from build123d import *

# Parameters (mm, degrees)
SALIENTE_EXTRUIR1_DEPTH  = 12
CROQUIS2_W               = 12.5
CROQUIS2_H               = 16.5
CROQUIS2_W_2             = 9.5
CROQUIS2_H_2             = 13.5
SALIENTE_EXTRUIR2_DEPTH  = 2
SALIENTE_EXTRUIR4_DEPTH  = 11
CROQUIS4_R               = 1.6
CORTAR_EXTRUIR1_DEPTH    = 2.5
CROQUIS5_W               = 17.29289048
CROQUIS5_H               = 2.276098228
CROQUIS5_W_2             = 23.449996424
CROQUIS5_H_2             = 5.821617307
CORTAR_EXTRUIR2_DEPTH    = 2
SALIENTE_EXTRUIR5_DEPTH  = 3
CROQUIS7_W               = 60
CROQUIS7_H               = 12
SALIENTE_EXTRUIR6_DEPTH  = 3
CORTAR_EXTRUIR3_DEPTH    = 42
VACIADO4_START           = -15.778481013
VACIADO4_DEPTH           = 39
VACIADO4_2_OUTLINE_W     = 28
VACIADO4_2_OUTLINE_H     = 9
VACIADO4_2_DEPTH         = 4
VACIADO4_START_2         = 19.221518987
VACIADO4_3_OUTLINE_W     = 28
VACIADO4_3_OUTLINE_H     = 9
VACIADO4_3_DEPTH         = 4
VACIADO4_START_3         = -3.938481013
VACIADO4_4_OUTLINE_W     = 9.5
VACIADO4_4_OUTLINE_H     = 1.5
VACIADO4_4_DEPTH         = 13.5
REDONDEO2_R              = 4
REDONDEO3_R              = 4
CROQUIS10_W              = 2.5
CROQUIS10_H              = 7
SALIENTE_EXTRUIR8_DEPTH  = 24
CROQUIS11_R              = 1.65
CORTAR_EXTRUIR4_DEPTH    = 2.5
CROQUIS14_R              = 1.6
SALIENTE_EXTRUIR10_DEPTH = 0.5
CROQUIS15_W              = 28.276285021
CROQUIS15_H              = 42
CORTAR_EXTRUIR5_DEPTH    = 12
CROQUIS16_W              = 42
CROQUIS16_H              = 12
SALIENTE_EXTRUIR11_DEPTH = 2
CORTAR_EXTRUIR6_DEPTH    = 2.5
CROQUIS19_W              = 18.223714979
CROQUIS19_H              = 1.5
SALIENTE_EXTRUIR16_DEPTH = 9
REDONDEO4_R              = 2
REDONDEO5_R              = 2
REDONDEO6_R              = 2


with BuildPart() as part:
    # Croquis1 → Saliente-Extruir1 (new body)
    with BuildSketch(Plane(origin=(0, 0, 0), x_dir=(1, 0, 0), z_dir=(0, 1, 0))):
        Polygon((30.683544304, -17.721518987), (30.683544304, -21.721518987), (-29.316455696, -21.721518987), (-29.316455696, 14.278481013), (30.683544304, 14.278481013), (30.683544304, 10.278481013), (2.683544304, 10.278481013), (2.683544304, -17.721518987), align=None)
    extrude(amount=SALIENTE_EXTRUIR1_DEPTH)

    # Croquis2 → Saliente-Extruir2 (add)
    with BuildSketch(Plane(origin=(0, 12, 0), x_dir=(1, 0, 0), z_dir=(0, 1, 0))):
        with Locations((-21.066455696, -2.811518987)):
            Rectangle(CROQUIS2_W, CROQUIS2_H)
        with Locations((-21.066455696, -2.811518987)):
            Rectangle(CROQUIS2_W_2, CROQUIS2_H_2, mode=Mode.SUBTRACT)
    extrude(amount=SALIENTE_EXTRUIR2_DEPTH)

    # Croquis3 → Saliente-Extruir4 (add)
    with BuildSketch(Plane(origin=(0, 12, 0), x_dir=(1, 0, 0), z_dir=(0, 1, 0))):
        Polygon((-7.816455696, -12.741518987), (-7.816455696, -41.560532566), (-7.816455696, -45.664219129), (-9.816455696, -45.664219129), (-9.816455696, -41.560532566), (-9.816455696, -12.741518987), align=None)
    extrude(amount=SALIENTE_EXTRUIR4_DEPTH)

    # Croquis4 → Cortar-Extruir1 (cut)
    with BuildSketch(Plane.ZY.offset(9.816455696)):
        with Locations((40.551518987, 19.507537468)):
            Circle(CROQUIS4_R)
    extrude(amount=-CORTAR_EXTRUIR1_DEPTH, mode=Mode.SUBTRACT)

    # Croquis5 → Cortar-Extruir2 (cut)
    with BuildSketch(Plane.ZY.offset(9.816455696)):
        with Locations((37.017773889, 13.138049114)):
            Rectangle(CROQUIS5_W, CROQUIS5_H)
        with Locations((24.466517199, 20.089191347)):
            Rectangle(CROQUIS5_W_2, CROQUIS5_H_2)
    extrude(amount=-CORTAR_EXTRUIR2_DEPTH, mode=Mode.SUBTRACT)

    # Croquis6 → Saliente-Extruir5 (add)
    with BuildSketch(Plane.XY.offset(21.721518987)):
        Polygon((-29.316455696, 0), (30.683544304, 0), (30.683544304, 12), (-7.816455696, 12), (-9.816455696, 12), (-29.316455696, 12), align=None)
    extrude(amount=SALIENTE_EXTRUIR5_DEPTH)

    # Croquis7 → Saliente-Extruir6 (add)
    with BuildSketch(Plane(origin=(0, 0, -14.278481013), x_dir=(-1, 0, 0), z_dir=(0, 0, -1))):
        with Locations((-0.683544304, 6)):
            Rectangle(CROQUIS7_W, CROQUIS7_H)
    extrude(amount=SALIENTE_EXTRUIR6_DEPTH)

    # Croquis8 → Cortar-Extruir3 (cut)
    with BuildSketch(Plane.XY.offset(24.721518987)):
        with BuildLine():
            Line((-29.316455696, 0), (-18.316455696, 0))
            ThreePointArc((-18.316455696, 0), (-26.094630289, 3.221825407), (-29.316455696, 11))
            Line((-29.316455696, 11), (-29.316455696, 0))
        make_face()
    extrude(amount=-CORTAR_EXTRUIR3_DEPTH, mode=Mode.SUBTRACT)

    # Vaciado4: read off the stored shape, not the designer's step
    # Vaciado4 outline → Vaciado4 (cut)
    with BuildSketch(Plane.XY.offset(VACIADO4_START)):
        with BuildLine():
            Line((1.183544304, 10.5), (-27.803288677, 10.5))
            ThreePointArc((-27.803288677, 10.5), (-24.854804112, 4.107975624), (-18.316455696, 1.5))
            Line((-18.316455696, 1.5), (1.183544304, 1.5))
            Line((1.183544304, 1.5), (1.183544304, 10.5))
        make_face()
    extrude(amount=VACIADO4_DEPTH, mode=Mode.SUBTRACT)

    # Vaciado4 2 outline → Vaciado4 2 (cut)
    with BuildSketch(Plane.XY.offset(VACIADO4_START)):
        with Locations((15.183544304, 6)):
            Rectangle(VACIADO4_2_OUTLINE_W, VACIADO4_2_OUTLINE_H)
    extrude(amount=VACIADO4_2_DEPTH, mode=Mode.SUBTRACT)

    # Vaciado4 3 outline → Vaciado4 3 (cut)
    with BuildSketch(Plane.XY.offset(VACIADO4_START_2)):
        with Locations((15.183544304, 6)):
            Rectangle(VACIADO4_3_OUTLINE_W, VACIADO4_3_OUTLINE_H)
    extrude(amount=VACIADO4_3_DEPTH, mode=Mode.SUBTRACT)

    # Vaciado4 4 outline → Vaciado4 4 (cut)
    with BuildSketch(Plane.XY.offset(VACIADO4_START_3)):
        with Locations((-21.066455696, 11.25)):
            Rectangle(VACIADO4_4_OUTLINE_W, VACIADO4_4_OUTLINE_H)
    extrude(amount=VACIADO4_4_DEPTH, mode=Mode.SUBTRACT)

    # Redondeo2
    # the kernel refuses this fillet: 4 mm, written as the material it adds along each edge
    with BuildSketch(Plane(origin=(-9.816455696, 12, 24.721518987), x_dir=(0, -1, 0), z_dir=(1, 0, 0))) as redondeo2_piece_1:
        with BuildLine():
            CenterArc((3.984641355, -4), REDONDEO2_R, 90, 84.977462971)
            Line((0, -3.649809662), (0, 0))
            Line((0, 0), (3.984641355, 0))
        make_face()
    extrude(amount=2)
    with BuildSketch(Plane(origin=(-9.816455696, 14.276098228, 28.371328649), x_dir=(0, 0, 1), z_dir=(1, 0, 0))) as redondeo2_piece_2:
        with BuildLine():
            CenterArc((3.609454623, 4), REDONDEO2_R, 205.52948015, 64.47051985)
            Line((0, 2.276098228), (0, 0))
            Line((0, 0), (3.609454623, 0))
        make_face()
    extrude(amount=2)
    with BuildSketch(Plane(origin=(-9.816455696, 17.178382693, 36.191515411), x_dir=(0, 0, -1), z_dir=(1, 0, 0))) as redondeo2_piece_3:
        with BuildLine():
            CenterArc((REDONDEO2_R, REDONDEO2_R), REDONDEO2_R, 180, 90)
            Line((0, REDONDEO2_R), (0, 0))
            Line((0, 0), (REDONDEO2_R, 0))
        make_face()
    extrude(amount=2)
    # the kernel refuses this fillet: 4 mm, written as the material it takes off along each edge
    with BuildSketch(Plane(origin=(-19.816455696, 17.178382693, 12.741518987), x_dir=(0, 0, 1), z_dir=(1, 0, 0))) as redondeo2_2_piece_1:
        with BuildLine():
            CenterArc((REDONDEO2_R, REDONDEO2_R), REDONDEO2_R, 180, 90)
            Line((0, REDONDEO2_R), (0, 0))
            Line((0, 0), (REDONDEO2_R, 0))
        make_face()
    extrude(amount=22, mode=Mode.SUBTRACT)

    # Redondeo3
    redondeo3_edges = [part.edges().sort_by_distance(p)[0] for p in [
        (-8.816455696, 23, 45.664219129),
        (-8.816455696, 14.276098228, 45.664219129),
    ]]
    fillet(redondeo3_edges, radius=REDONDEO3_R)

    # Croquis10 → Saliente-Extruir8 (add)
    with BuildSketch(Plane(origin=(0, 12, 0), x_dir=(1, 0, 0), z_dir=(0, 1, 0))):
        with Locations((-15.066455696, 10.278481013)):
            Rectangle(CROQUIS10_W, CROQUIS10_H)
    extrude(amount=SALIENTE_EXTRUIR8_DEPTH)

    # Croquis11 → Cortar-Extruir4 (cut)
    with BuildSketch(Plane.ZY.offset(16.316455696)):
        with Locations((-10.278481013, 32.003262859)):
            Circle(CROQUIS11_R)
    extrude(amount=-CORTAR_EXTRUIR4_DEPTH, mode=Mode.SUBTRACT)

    # Croquis14 → Saliente-Extruir10 (add)
    with BuildSketch(Plane(origin=(-7.816455696, 0, 0), x_dir=(0, 0, -1), z_dir=(1, 0, 0))):
        with BuildLine():
            Line((-36.191515411, 23), (-41.664219129, 23))
            ThreePointArc((-41.664219129, 23), (-44.492646254, 21.828427125), (-45.664219129, 19))
            Line((-45.664219129, 19), (-45.664219129, 18.276098228))
            ThreePointArc((-45.664219129, 18.276098228), (-44.492646254, 15.447671103), (-41.664219129, 14.276098228))
            Line((-41.664219129, 14.276098228), (-31.980783273, 14.276098228))
            ThreePointArc((-31.980783273, 14.276098228), (-29.847195577, 13.659558519), (-28.371328649, 12))
            ThreePointArc((-28.371328649, 12), (-25.771878217, 10.717139414), (-24.721518987, 8.015358645))
            Line((-24.721518987, 8.015358645), (-24.721518987, 12))
            Line((-24.721518987, 12), (-12.741518987, 12))
            Line((-12.741518987, 12), (-12.741518987, 13.178382693))
            ThreePointArc((-12.741518987, 13.178382693), (-13.913091863, 16.006809817), (-16.741518987, 17.178382693))
            Line((-16.741518987, 17.178382693), (-32.191515411, 17.178382693))
            ThreePointArc((-32.191515411, 17.178382693), (-35.019942535, 18.349955568), (-36.191515411, 21.178382693))
            Line((-36.191515411, 21.178382693), (-36.191515411, 23))
        make_face()
        with Locations(Location((-40.551518987, 19.507537468, 0), (0, 0, 180))):
            Circle(CROQUIS14_R, mode=Mode.SUBTRACT)
    extrude(amount=SALIENTE_EXTRUIR10_DEPTH)

    # Croquis15 → Cortar-Extruir5 (cut)
    with BuildSketch(Plane(origin=(0, 12, 0), x_dir=(1, 0, 0), z_dir=(0, 1, 0))):
        with Locations((16.545401794, -3.721518987)):
            Rectangle(CROQUIS15_W, CROQUIS15_H)
    extrude(amount=-CORTAR_EXTRUIR5_DEPTH, mode=Mode.SUBTRACT)

    # Croquis16 → Saliente-Extruir11 (add)
    with BuildSketch(Plane(origin=(2.407259283, 0, 0), x_dir=(0, 0, -1), z_dir=(1, 0, 0))):
        with Locations((-3.721518987, 6)):
            Rectangle(CROQUIS16_W, CROQUIS16_H)
    extrude(amount=-SALIENTE_EXTRUIR11_DEPTH)

    # Croquis18 → Cortar-Extruir6 (cut)
    with BuildSketch(Plane(origin=(2.407259283, 0, 0), x_dir=(0, 0, -1), z_dir=(1, 0, 0))):
        with BuildLine():
            Line((-20.721518987, 5.5), (13.278481013, 5.5))
            ThreePointArc((13.278481013, 5.5), (14.692694575, 4.914213562), (15.278481013, 3.5))
            Line((15.278481013, 3.5), (15.278481013, 3.3))
            ThreePointArc((15.278481013, 3.3), (14.692694575, 1.885786438), (13.278481013, 1.3))
            Line((13.278481013, 1.3), (-20.721518987, 1.3))
            ThreePointArc((-20.721518987, 1.3), (-22.13573255, 1.885786438), (-22.721518987, 3.3))
            Line((-22.721518987, 3.3), (-22.721518987, 3.5))
            ThreePointArc((-22.721518987, 3.5), (-22.13573255, 4.914213562), (-20.721518987, 5.5))
        make_face()
    extrude(amount=-CORTAR_EXTRUIR6_DEPTH, mode=Mode.SUBTRACT)

    # Croquis19 → Saliente-Extruir16 (add)
    with BuildSketch(Plane(origin=(0, 1.5, 0), x_dir=(1, 0, 0), z_dir=(0, 1, 0))):
        with Locations((-9.204598207, -17.846071371)):
            Rectangle(CROQUIS19_W, CROQUIS19_H)
        with Locations((-9.224216979, -4.59531752)):
            Rectangle(CROQUIS19_W, CROQUIS19_H)
        with Locations((-9.175696895, 9.179239743)):
            Rectangle(CROQUIS19_W, CROQUIS19_H)
    extrude(amount=SALIENTE_EXTRUIR16_DEPTH)

    # Redondeo4
    # the kernel refuses this fillet: 2 mm, written as the material it takes off along each edge
    with BuildSketch(Plane(origin=(2.407259283, 12, -22.278481013), x_dir=(-1, 0, 0), z_dir=(0, 0, 1))) as redondeo4_piece_1:
        with BuildLine():
            CenterArc((REDONDEO4_R, REDONDEO4_R), REDONDEO4_R, 180, 90)
            Line((0, REDONDEO4_R), (0, 0))
            Line((0, 0), (REDONDEO4_R, 0))
        make_face()
    extrude(amount=52, mode=Mode.SUBTRACT)
    with BuildSketch(Plane(origin=(2.407259283, 17, 24.721518987), x_dir=(-1, 0, 0), z_dir=(0, -1, 0)), Plane(origin=(2.407259283, 17, -17.278481013), x_dir=(0, 0, 1), z_dir=(0, -1, 0))) as redondeo4_piece_2:
        with BuildLine():
            CenterArc((REDONDEO4_R, REDONDEO4_R), REDONDEO4_R, 180, 90)
            Line((0, REDONDEO4_R), (0, 0))
            Line((0, 0), (REDONDEO4_R, 0))
        make_face()
    extrude(amount=22, mode=Mode.SUBTRACT)

    # Redondeo5
    redondeo5_edges = [part.edges().sort_by_distance(p)[0] for p in [
        (-15.066455696, 36, -13.778481013),
        (-15.066455696, 36, -6.778481013),
    ]]
    fillet(redondeo5_edges, radius=REDONDEO5_R)

    # Redondeo6
    redondeo6_edges = [part.edges().sort_by_distance(p)[0] for p in [
        (-13.816455696, 12, -10.278481013),
        (-15.066455696, 12, -13.778481013),
        (-16.316455696, 12, -10.278481013),
    ]]
    fillet(redondeo6_edges, radius=REDONDEO6_R)


solid = part.part
Design review of the part built by this model. Coordinates are the model's own, in mm. A direction names the side the tool comes from. Coordinates: 2 decimals unless noted, no trailing zeros. Loops run counter-clockwise (first coordinate to the right, second up) from the corner with the lowest first, then second, coordinate; pieces in that order, holes last.
Item 1: For faces 1 (the flat face through (-21, 13, -5.438)), 2 (the flat face through (-9, 14.276, 37)), 3 (the flat face through (-21, 12, -3.938)), list the 3-axis set-ups (+Z, -Z, +X, -X, +Y, -Y) from which the entire face can be reached by the end or side of a thin tool; tool diameter is ignored.
Completed:
face 1: +X, -X, +Y
face 2: +Z, +X, -X, -Y
face 3: +Y
Item 2: Draft analysis for pull direction Z (two halves, no side actions). For faces 4 (the flat face through (-9, 6, -8.429)), 5 (the cylindrical face through (1.837, 6.084, 24.12)), 6 (the cylindrical face through (1.806, 6.084, -16.708)), state which applies: pulls with the +Z half, pulls with the -Z half, needs draft (parallel to the pull), parting line crosses it, or undercut.
Completed:
face 4: undercut
face 5: pulls with the +Z half
face 6: pulls with the -Z half
Item 3: Add section A-A (x = -10.5). Write out the cut boundary in (y, z), and give its area (4 significant figures).
Completed:
outline: (0, -17.28) - (12, -17.28) - (12, 24.72) - (0, 24.72) - close; hole (1.5, -15.78) - (10.5, -15.78) - (10.5, -9.93) - (1.5, -9.93) - close; hole (1.5, -8.43) - (10.5, -8.43) - (10.5, 3.85) - (1.5, 3.85) - close; hole (1.5, 5.35) - (10.5, 5.35) - (10.5, 17.1) - (1.5, 17.1) - close; hole (1.5, 18.6) - (10.5, 18.6) - (10.5, 23.22) - (1.5, 23.22) - close
area: 193.5 mm2
Item 4: Add section D-D (x = -19). Write out the cut boundary in (y, z).
Completed:
outline: (0.02, -17.28) - (12, -17.28) - (12, -5.44) - (14, -5.44) - (14, -3.94) - (10.5, -3.94) - (10.5, -15.78) - (1.52, -15.78) - (1.52, 23.22) - (10.5, 23.22) - (10.5, 9.56) - (14, 9.56) - (14, 11.06) - (12, 11.06) - (12, 24.72) - (0.02, 24.72) - close
Item 5: Add section B-B (z = 40.5). Write out the cut boundary in (x, y), and give its area (3 significant figures).
Completed:
outline: (-9.82, 14.28) - (-7.32, 14.28) - (-7.32, 17.91) - (-9.82, 17.91) - close; (-9.82, 21.11) - (-7.32, 21.11) - (-7.32, 23) - (-9.82, 23) - close
area: 13.8 mm2
Item 6: Wall thickness on L1, parallel to Z at x = -16, y = 7.5; L2, parallel to Y at x = -1, z = -6; L3, parallel to X at y = 9.5, z = 18: over which ranges is each line inside the solid? List them lowest first.
Completed:
L1: z = -17.28 to -15.78, -9.93 to -8.43, 3.85 to 5.35, 17.1 to 18.6, 23.22 to 24.72
L2: y = 0 to 1.5, 10.5 to 12
L3: x = -29.21 to -27.7, -18.32 to -0.09, 0.41 to 2.41
Item 7: Clearance check with flat-ended pins moving along their axes: pin 1 (0.6 mm diameter, centred on x = -9, y = 13, fed in from -Z); pin 2 (1.5 mm diameter, centred on x = -11.5, z = 34.5, fed in from -Y); pin 3 (4 mm diameter, centred on y = 19.51, z = 40.55, fed in from -X); pin 4 (1 mm diameter, centred on y = 9.5, z = 15, fed in from -X). State where each tip first meets the part, or that it passes through.
Completed:
pin 1: stops at z = 12.74
pin 2: passes through
pin 3: stops at x = -9.82
pin 4: stops at x = -29.27
Item 8: Add section C-C (z = 12). Write out the cut boundary in (x, y), and give its area (3 significant figures).
Completed:
outline: (-29.32, 11) arc R11 ccw to (-18.32, 0) - (2.41, 0) - (2.41, 1.3) - (-0.09, 1.3) - (-0.09, 1.5) - (-18.32, 1.5) arc R9.5 cw to (-27.8, 10.5) - (0.41, 10.5) - (0.41, 5.5) - (2.41, 5.5) - (2.41, 10) arc R2 ccw to (0.41, 12) - (-29.32, 12) - close
area: 111 mm2
